from build123d import *

# Parameters (mm, degrees)
SKETCH1_R                = 20
BOSS_EXTRUDE1_DEPTH      = 50
SKETCH2_R                = 40
BOSS_EXTRUDE2_DEPTH      = 5
CHAMFER1_SIZE            = 2
SKETCH3_R                = 2.5
CUT_EXTRUDE1_DEPTH       = 120.268604419
CIRPATTERN1_COUNT        = 6
FILLET4_R                = 3
MIRROR1_COPY_1_SKETCH_R  = 2.5
MIRROR1_COPY_1_DEPTH     = 120.268604419
MIRROR1_COPY_2_SKETCH_R  = 2.5
MIRROR1_COPY_2_DEPTH     = 120.268604419
MIRROR1_COPY_3_SKETCH_R  = 2.5
MIRROR1_COPY_3_DEPTH     = 120.268604419
MIRROR1_COPY_4_SKETCH_R  = 2.5
MIRROR1_COPY_4_DEPTH     = 120.268604419
MIRROR1_COPY_5_SKETCH_R  = 2.5
MIRROR1_COPY_5_DEPTH     = 120.268604419
CHAMFER1_OF_MIRROR1_SIZE = 2
FILLET4_OF_MIRROR1_R     = 3


with BuildPart() as part:
    # Sketch1 → Boss-Extrude1 (new, symmetric)
    with BuildSketch(Plane(origin=(0, 0, 0), x_dir=(1, 0, 0), z_dir=(0, 1, 0))):
        with Locations(Location((0, 0, 0), (0, 0, 270))):
            Circle(SKETCH1_R)
    extrude(amount=BOSS_EXTRUDE1_DEPTH, both=True)

    # Sketch2 → Boss-Extrude2 (add)
    with BuildSketch(Plane(origin=(0, 50, 0), x_dir=(1, 0, 0), z_dir=(0, 1, 0))):
        with Locations(Location((0, 0, 0), (0, 0, 270))):
            Circle(SKETCH2_R)
    boss_extrude2 = extrude(amount=BOSS_EXTRUDE2_DEPTH)

    # Chamfer1
    chamfer1_edges = [part.edges().sort_by_distance(p)[0] for p in [
        (0, 55, -40),
    ]]
    chamfer(chamfer1_edges, length=CHAMFER1_SIZE)

    # Sketch3 → Cut-Extrude1 (cut, through all)
    with BuildSketch(Plane(origin=(0, 55, 0), x_dir=(1, 0, 0), z_dir=(0, 1, 0))):
        with Locations(Location((0, 29, 0), (0, 0, 270))):
            Circle(SKETCH3_R)
    cut_extrude1 = extrude(amount=-CUT_EXTRUDE1_DEPTH, mode=Mode.SUBTRACT)

    # CirPattern1: Cut-Extrude1 ×6 about axis
    cirpattern1_axis = Axis((0, 0, 0), (0, 1, 0))
    for i in range(1, CIRPATTERN1_COUNT):
        add(cut_extrude1.rotate(cirpattern1_axis, i * 360 / CIRPATTERN1_COUNT), mode=Mode.SUBTRACT)

    # Fillet4
    fillet4_edges = [part.edges().sort_by_distance(p)[0] for p in [
        (0, 50, -20),
    ]]
    fillet(fillet4_edges, radius=FILLET4_R)

    # Sketch5 → CBORE for #12 Binding Head Machine Screw1 (revolve, cut)
    with BuildSketch(Plane(origin=(0, 55, 0), x_dir=(0, 0, 1), z_dir=(1, 0, 0))):
        Polygon((0, 0), (0, 110), (2.8956, 110), (2.8956, 3.5814), (5.95376, 3.5814), (5.95376, 0.635), (6.58876, 0), align=None)
    cbore_for_12_binding_head_machine_screw = revolve(axis=Axis((0, 61.35, 0), (0, -1, 0)), mode=Mode.SUBTRACT)

    # Mirror1: Boss-Extrude2, Cut-Extrude1, CBORE for #12 Binding Head Machine Screw1 across plane
    add(boss_extrude2.mirror(Plane.ZX))
    add(cut_extrude1.mirror(Plane.ZX), mode=Mode.SUBTRACT)
    add(cbore_for_12_binding_head_machine_screw.mirror(Plane.ZX), mode=Mode.SUBTRACT)

    # Mirror1 copy 1 sketch → Mirror1 copy 1 (cut, through all)
    with BuildSketch(Plane(origin=(0, -55, 0), x_dir=(0.5000000000000001, 0, -0.8660254037844386), z_dir=(0, -1, 0))):
        with Locations((0, -29)):
            Circle(MIRROR1_COPY_1_SKETCH_R)
    extrude(amount=-MIRROR1_COPY_1_DEPTH, mode=Mode.SUBTRACT)

    # Mirror1 copy 2 sketch → Mirror1 copy 2 (cut, through all)
    with BuildSketch(Plane(origin=(0, -55, 0), x_dir=(-0.4999999999999998, 0, -0.8660254037844387), z_dir=(0, -1, 0))):
        with Locations((0, -29)):
            Circle(MIRROR1_COPY_2_SKETCH_R)
    extrude(amount=-MIRROR1_COPY_2_DEPTH, mode=Mode.SUBTRACT)

    # Mirror1 copy 3 sketch → Mirror1 copy 3 (cut, through all)
    with BuildSketch(Plane(origin=(0, -55, 0), x_dir=(-1, 0, 0), z_dir=(0, -1, 0))):
        with Locations((0, -29)):
            Circle(MIRROR1_COPY_3_SKETCH_R)
    extrude(amount=-MIRROR1_COPY_3_DEPTH, mode=Mode.SUBTRACT)

    # Mirror1 copy 4 sketch → Mirror1 copy 4 (cut, through all)
    with BuildSketch(Plane(origin=(0, -55, 0), x_dir=(-0.5000000000000004, 0, 0.8660254037844384), z_dir=(0, -1, 0))):
        with Locations((0, -29)):
            Circle(MIRROR1_COPY_4_SKETCH_R)
    extrude(amount=-MIRROR1_COPY_4_DEPTH, mode=Mode.SUBTRACT)

    # Mirror1 copy 5 sketch → Mirror1 copy 5 (cut, through all)
    with BuildSketch(Plane(origin=(0, -55, 0), x_dir=(0.5000000000000001, 0, 0.8660254037844386), z_dir=(0, -1, 0))):
        with Locations((0, -29)):
            Circle(MIRROR1_COPY_5_SKETCH_R)
    extrude(amount=-MIRROR1_COPY_5_DEPTH, mode=Mode.SUBTRACT)

    # Chamfer1 of Mirror1
    chamfer1_of_mirror1_edges = [part.edges().sort_by_distance(p)[0] for p in [
        (0, -55, -40),
    ]]
    chamfer(chamfer1_of_mirror1_edges, length=CHAMFER1_OF_MIRROR1_SIZE)

    # Fillet4 of Mirror1
    fillet4_of_mirror1_edges = [part.edges().sort_by_distance(p)[0] for p in [
        (0, -50, -20),
    ]]
    fillet(fillet4_of_mirror1_edges, radius=FILLET4_OF_MIRROR1_R)


solid = part.part
Part model, mm, in its own coordinate system. A direction names the side the tool comes from. Coordinates: 2 decimals unless noted, no trailing zeros. Order: outer loops, then holes, each group sorted by start corner. A loop starts at its lowest first (then second) coordinate and runs counter-clockwise, first axis right, second up. Notation, with made-up numbers: M -5.75,-30.5 L 21.25,-30.5 A29 ccw 21.25,-4.5 Z; hole C 57.25,-38.5 d1. An arc over 180 degrees is marked long. Use a Markdown table: item, result.
(1) Cut at A-A on x = 0. State how many separate pieces and enclosed holes the cut face has, then the cut area to 3 significant figures.
A:
| item | result |
|---|---|
| separate pieces | 6 |
| enclosed holes | 0 |
| area | 4,020 mm^2 |
(2) Probe L1, parallel to X at y = 52, z = 14; L2, parallel to X at y = 51.55, z = 14.5; L3, parallel to Y at x = 34, z = 3. List the from-to ranges inside material, lowest first.
A:
| item | result |
|---|---|
| L1 | x = -37.47 to -27.56, -22.67 to 22.67, 27.56 to 37.47 |
| L2 | x = -37.28 to -27.61, -22.61 to 22.61, 27.61 to 37.28 |
| L3 | y = -55 to -50, 50 to 55 |
(3) Tool access for faces 1 (the flat face through (-17, 50, 17)), 2 (the flat face through (-1, 51.419, -3)), 3 (the flat face through (-1, -51.419, -3)): list every direction of +Z, -Z, +X, -X, +Y, -Y with a clear straight run to the whole face (end or side of a thin tool).
A:
| item | result |
|---|---|
| face 1 | none |
| face 2 | +Y |
| face 3 | -Y |
(4) Cut at B-B on y = 14.5. Write the cut outline in (x, z), then the cut area to 3 significant figures.
A:
| item | result |
|---|---|
| outline | C 0,0 d40; hole C 0,0 d5.79 |
| area | 1,230 mm^2 |
(5) Flat gauge pins, fed straight in: pin 1 (9.5 mm diameter, centred on x = 0, z = 0, fed in from -Y); pin 2 (6 mm diameter, centred on x = -25.11, z = -14.5, fed in from -Y); pin 3 (1.5 mm diameter, centred on x = -2, y = -0.5, fed in from -Z); pin 4 (9.5 mm diameter, centred on x = 0, z = 0, fed in from +Y). Where does each tip first touch, or does it go through?
A:
| item | result |
|---|---|
| pin 1 | stops at y = -51.42 |
| pin 2 | stops at y = -55 |
| pin 3 | stops at z = -19.96 |
| pin 4 | stops at y = 51.42 |
(6) Pull direction X, two halves, no side cores. Call faces 4 (the cylindrical face through (-0.1, 52.5, 31.5)), 5 (the cylindrical face through (-19.524, 0.658, -4.336)), 6 (the flat face through (-8, 55, -1)), 7 (the cylindrical face through (0.1, -52.5, -31.5)): released by +X, released by -X, zero draft, split by the parting line, or undercut.
A:
| item | result |
|---|---|
| face 4 | undercut |
| face 5 | split by the parting line |
| face 6 | zero draft |
| face 7 | undercut |
